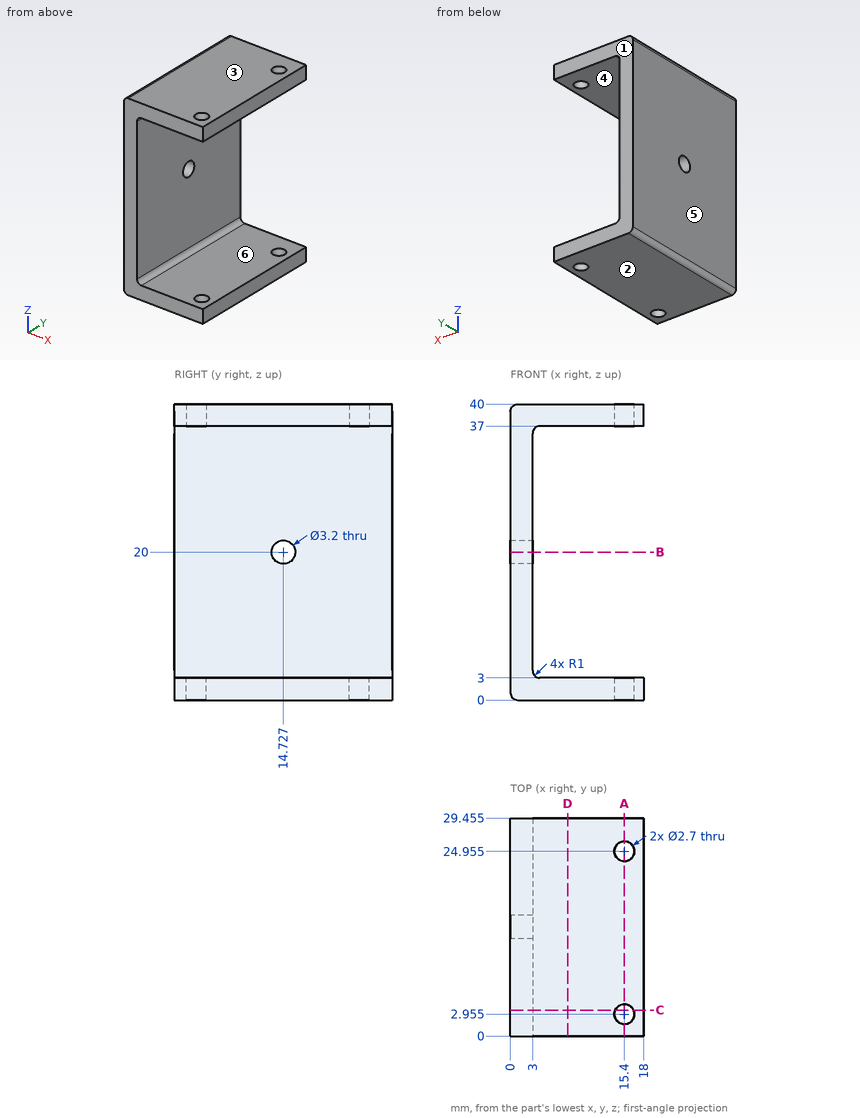
Source: three-view drawing plus pictorial views. Frame: mm from the lowest corner of the part. A direction names the side the tool comes from. Give positions to 0.01 mm unless a question says otherwise; leave off trailing zeros. Order: outer loops, then holes, each group sorted by start corner. A loop starts at its lowest first (then second) coordinate and runs counter-clockwise, first axis right, second up.
1. Section B-B on z = 20. Return the cut outline in (x, y) (1 decimal).
Derived:
outline: (0, 0) - (3, 0) - (3, 13.1) - (0, 13.1) - close; (0, 16.3) - (3, 16.3) - (3, 29.5) - (0, 29.5) - close
2. Pin query (flat end, axial travel): pin 1 (2 mm diameter, centred on x = 15.4, y = 2.95, fed in from -Z); pin 2 (6 mm diameter, centred on y = 14, z = 13.5, fed in from +X). Return the tip coordinate at first contact, or that it passes through.
Derived:
pin 1: passes through
pin 2: stops at x = 3
3. Section D-D on x = 7.75. Return the cut outline in (y, z) (1 decimal).
Derived:
outline: (0, 0) - (29.5, 0) - (29.5, 3) - (0, 3) - close; (0, 37) - (29.5, 37) - (29.5, 40) - (0, 40) - close
4. Material intervals for L1, parallel to Y at x = 15.4, z = 0.9 (1 decimal); L2, parallel to Z at x = 7, y = 22; L3, parallel to Y at x = 0.95, z = 20 (1 decimal), sorted ascending.
Derived:
L1: y = 0 to 1.6, 4.3 to 23.6, 26.3 to 29.5
L2: z = 0 to 3, 37 to 40
L3: y = 0 to 13.1, 16.3 to 29.5
5. Mould query, pull axis Z, two halves, no side actions, for the marked faces 1, 2, 3 and 4. Classes: released by +Z, released by -Z, zero draft, split by the parting line, or undercut.
Derived:
face 1: zero draft
face 2: released by -Z
face 3: released by +Z
face 4: undercut
6. Section C-C on y = 3.5. Return the cut outline in (x, z) (1 decimal).
Derived:
outline: (0, 1) arc R1 ccw to (1, 0) - (14.2, 0) - (14.2, 3) - (4, 3) arc R1 cw to (3, 4) - (3, 36) arc R1 cw to (4, 37) - (14.2, 37) - (14.2, 40) - (1, 40) arc R1 ccw to (0, 39) - close; (16.6, 0) - (18, 0) - (18, 3) - (16.6, 3) - close; (16.6, 37) - (18, 37) - (18, 40) - (16.6, 40) - close
7. Section A-A on x = 15.4. Return the cut outline in (y, z) (1 decimal).
Derived:
outline: (0, 0) - (1.6, 0) - (1.6, 3) - (0, 3) - close; (0, 37) - (1.6, 37) - (1.6, 40) - (0, 40) - close; (4.3, 0) - (23.6, 0) - (23.6, 3) - (4.3, 3) - close; (4.3, 37) - (23.6, 37) - (23.6, 40) - (4.3, 40) - close; (26.3, 0) - (29.5, 0) - (29.5, 3) - (26.3, 3) - close; (26.3, 37) - (29.5, 37) - (29.5, 40) - (26.3, 40) - close
8. Reachability of the marked faces 5 and 6 from +Z, -Z, +X, -X, +Y, -Y: full face, straight path, thin tool, end or side. Return the list, or none.
Derived:
face 5: +Z, -Z, -X, +Y, -Y
face 6: +X, +Y, -Y
